Source: three-view drawing plus pictorial views. Frame: mm from the lowest corner of the part. A direction names the side the tool comes from. Round coordinates to 2 decimals unless told otherwise and drop trailing zeros. Loops run counter-clockwise (first coordinate to the right, second up) from the corner with the lowest first, then second, coordinate; pieces in that order, holes last. Notation, with made-up numbers: (-19.5, 88.5) -> (33.5, 88.5) arc R20 ccw to (33.5, 118.5) -> close; hole circle Ø1 at (-22, 60.25). An arc over 180 degrees is marked (long way). Return JSON: item names as keys, results as strings. Group by question number.
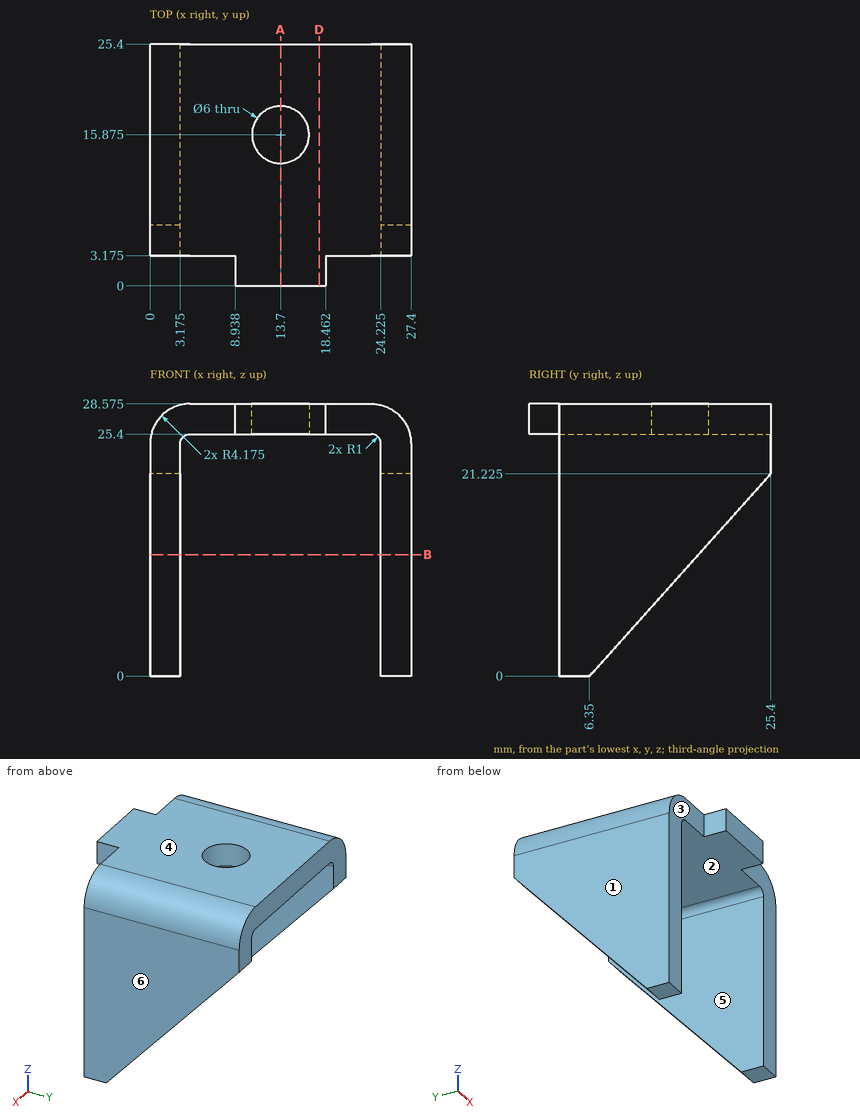
(1) Cut plane A-A (x = 13.7). Return loops of the section in (y, z) (1 decimal).
(2) Pin query (flat end, axial travel): pin 1 (4 mm diameter, centred on x = 7, z = 24.5, fed in from -Y) (1 decimal); pin 2 (1.6 mm diameter, centred on y = 2.5, z = 26.5, fed in from +X); pin 3 (1 mm diameter, centred on x = 14.5, y = 4.5, fed in from -Z); pin 4 (8 mm diameter, centred on x = 13.7, y = 15.875, fed in from +Z) (1 decimal). Return the tip coordinate at first contact, or that it passes through.
(3) Mould query, pull axis X, two halves, no side actions, for the marked faces 4, 5 and 6. Classes: released by +X, released by -X, zero draft, split by the parting line, or undercut.
(4) Cut plane D-D (x = 17.75). Return loops of the section in (y, z) (1 decimal).
(5) Set-up query: the marked faces 1, 2 and 3. Return all of +Z, -Z, +X, -X, +Y, -Y with unobstructed straight access to the full face (end or side cutting, diameter ignored); none if empty.
(6) Ray query, line 1 (Y direction, x = 13.7, z = 26.25) (1 decimal); line 2 (X direction, y = 4.5, z = 15.75) (1 decimal); line 3 (Z direction, x = 11, y = 1) (1 decimal). Return the intervals inside material, ascending.
(7) Cut plane B-B (z = 12.75). Return loops of the section in (x, y) (1 decimal).
Answers follow:
{
 "1": {"outline": "(0, 25.4) -> (12.9, 25.4) -> (12.9, 28.6) -> (0, 28.6) -> close; (18.9, 25.4) -> (25.4, 25.4) -> (25.4, 28.6) -> (18.9, 28.6) -> close"},
 "2": {"pin 1": "y = 3.2", "pin 2": "x = 27.05", "pin 3": "z = 25.4", "pin 4": "z = 28.6"},
 "3": {"face 4": "zero draft", "face 5": "undercut", "face 6": "released by +X"},
 "4": {"outline": "(0, 25.4) -> (25.4, 25.4) -> (25.4, 28.6) -> (0, 28.6) -> close"},
 "5": {"face 1": "+Z, -Z, -X, +Y, -Y", "face 2": "-Z, +Y, -Y", "face 3": "+Z, -Z, -X, -Y"},
 "6": {"line 1": "0 to 12.9, 18.9 to 25.4", "line 2": "0 to 3.2, 24.2 to 27.4", "line 3": "25.4 to 28.6"},
 "7": {"outline": "(0, 3.2) -> (3.2, 3.2) -> (3.2, 17.8) -> (0, 17.8) -> close; (24.2, 3.2) -> (27.4, 3.2) -> (27.4, 17.8) -> (24.2, 17.8) -> close"}
}
